Model file for the job. Use its own axes, mm. A direction names the side the tool comes from. Coordinates: 2 decimals unless noted, no trailing zeros. Order: outer loops, then holes, each group sorted by start corner. A loop starts at its lowest first (then second) coordinate and runs counter-clockwise, first axis right, second up. Notation, with made-up numbers: M -23.5,83 L 30.5,83 A23 cw 30.5,121 Z; hole C -11,57 d7. An arc over 180 degrees is marked long. Return JSON: item names as keys, results as strings.
```python
from build123d import *

# Parameters (mm, degrees)
F1_DEPTH = 9.525


with BuildPart() as f1:
    # F0 (on Top) → F1 (new body)
    with BuildSketch(Plane.XY):
        with BuildLine():
            Line((-10.026586, 12.900152), (-33.045336, 12.900152))
            Line((-33.045336, 12.900152), (-33.045336, 7.820152))
            Line((-33.045336, 7.820152), (-29.39147, 7.820152))
            ThreePointArc((-29.39147, 7.820152), (-26.85147, 10.360152), (-24.31147, 7.820152))
            Line((-24.31147, 7.820152), (5.271212, 7.820152))
            ThreePointArc((5.271212, 7.820152), (8.238203, 10.356891), (11.422657, 8.099163))
            Line((11.422657, 8.099163), (49.822164, 11.630152))
            Line((49.822164, 11.630152), (49.822164, 12.900152))
            Line((49.822164, 12.900152), (-8.121586, 12.900152))
            Line((-8.121586, 12.900152), (-8.121586, 11.312652))
            Line((-8.121586, 11.312652), (-10.026586, 11.312652))
            Line((-10.026586, 11.312652), (-10.026586, 12.900152))
        make_face()
    extrude(amount=F1_DEPTH)


solid = f1.part
```
Item 1: Saw through at C-C (x = 24). Write the cut outline in (y, z) (3 decimals).
Check result:
{"outline": "M 9.256,0 L 12.9,0 L 12.9,9.525 L 9.256,9.525 Z"}
Item 2: Saw through at B-B (z = 8). Write the cut outline in (x, y) (3 decimals), and give its area (3 significant figures).
Check result:
{"outline": "M -33.045,7.82 L -29.391,7.82 A2.54 cw -24.311,7.82 L 5.271,7.82 A3.175 cw 11.423,8.099 L 49.822,11.63 L 49.822,12.9 L -8.122,12.9 L -8.122,11.313 L -10.027,11.313 L -10.027,12.9 L -33.045,12.9 Z", "area": "317 mm2"}
Item 3: Pull direction X, two halves, no side cores. Call faces 1 (the flat face through (-33.045, 10, 5)), 2 (the flat face through (-9, 11.313, 5)), 3 (the flat face through (-1, 11, 9.525)): +X half, -X half, draft (parallel to the pull), parting line (faces both ways), or undercut.
Check result:
{"face 1": "-X half", "face 2": "undercut", "face 3": "draft"}
Item 4: Drop a flat-ended pin along its axis: pin 1 Ø1 at (x, z) = (34.5, 3) entering from -Y. Give the stop position or say it passes through.
Check result:
{"pin 1": "stops at y = 10.18"}
Item 5: 3-axis set-ups, long thin cutter, end or side, ignore diameter. For faces 4 (the flat face through (-8.122, 12, 5)), 5 (the flat face through (-21, 12.9, 5)): which of +Z, -Z, +X, -X, +Y, -Y reach the whole face in a straight line?
Check result:
{"face 4": "+Z, -Z, +Y", "face 5": "+Z, -Z, +X, -X, +Y"}
Item 6: Wall check: line 1 (X direction, y = 11.7, z = 1.75); line 2 (Y direction, x = 9, z = 9); line 3 (Y direction, x = -28, z = 1.5). Give the ranges that are in metal, low to high.
Check result:
{"line 1": "x = -33.05 to -10.03, -8.12 to 49.82", "line 2": "y = 10.3 to 12.9", "line 3": "y = 10.09 to 12.9"}
Item 7: Saw through at D-D (x = 13). Write the cut outline in (y, z) (3 decimals).
Check result:
{"outline": "M 8.244,0 L 12.9,0 L 12.9,9.525 L 8.244,9.525 Z"}
Item 8: Saw through at A-A (y = 9.2). Write the cut outline in (x, z) (3 decimals), and give its area (3 significant figures).
Check result:
{"outline": "M -33.045,0 L -28.984,0 L -28.984,9.525 L -33.045,9.525 Z; M -24.719,0 L 5.928,0 L 5.928,9.525 L -24.719,9.525 Z; M 10.836,0 L 23.394,0 L 23.394,9.525 L 10.836,9.525 Z", "area": "450 mm2"}
